Here's how the part is built. I have some questions about the finished solid (model axes, mm). A direction names the side the tool comes from. Give positions to 0.01 mm unless a question says otherwise; leave off trailing zeros. Write each loop counter-clockwise with the first axis right and the second up, starting at its lowest first coordinate (ties: lowest second). Pieces come first, ordered by that corner, then holes. Notation, with made-up numbers: (70, 34) - (95, 34) arc R27 ccw to (95, 53) - close; hole circle Ø1 at (80.25, 78.25). An arc over 180 degrees is marked (long way). Use one line per item in the form item = value. Start each with the question number.
from build123d import *

# Parameters (mm, degrees)
SKETCH1_W           = 40
SKETCH1_H           = 40
BOSS_EXTRUDE1_DEPTH = 50
SKETCH2_W           = 35
SKETCH2_H           = 35
CUT_EXTRUDE1_DEPTH  = 76.498344353
CUT_EXTRUDE2_DEPTH  = 76.498344353


with BuildPart() as part:
    # Sketch1 → Boss-Extrude1 (new body)
    with BuildSketch(Plane(origin=(0, 0, 0), x_dir=(1, 0, 0), z_dir=(0, 1, 0))):
        with Locations((20, 20)):
            Rectangle(SKETCH1_W, SKETCH1_H)
    extrude(amount=BOSS_EXTRUDE1_DEPTH)

    # Sketch2 → Cut-Extrude1 (cut, through all)
    with BuildSketch(Plane.XZ):
        with Locations((20, -20)):
            Rectangle(SKETCH2_W, SKETCH2_H)
    extrude(amount=-CUT_EXTRUDE1_DEPTH, mode=Mode.SUBTRACT)

    # Sketch3 → Cut-Extrude2 (cut, through all)
    with BuildSketch(Plane.ZY):
        Polygon((-40, 0), (0, 0), (-40, 14.558809371), align=None)
        Polygon((-40, 50), (0, 35.441190629), (0, 50), align=None)
    extrude(amount=-CUT_EXTRUDE2_DEPTH, mode=Mode.SUBTRACT)


solid = part.part
1. I want a section at A-A, the plane x = 5. List the corners of the cut face in (y, z) for me, then the cut area to 3 significant figures.
2. For faces 1 (the face through (37.5, 25, -20)), 2 (the face through (20, 32, -40)), which set-ups out of +Z, -Z, +X, -X, +Y, -Y let a thin tool reach every point of the face, with its end or its side?
3. I want a section at D-D, the plane y = 45.5. List the corners of the cut face in (x, z) for me.
4. Please list where these lines run through material, in increasing order: line 1 (X direction, y = 20, z = -8); line 2 (Z direction, x = 10.5, y = 23); line 3 (Z direction, x = 7, y = 5).
5. We'd pull the mould along X, two halves only. Please class faces 3 (the face through (2.129, 42.755, -20.093)), 4 (the face through (2.5, 25, -20)), 5 (the face through (40, 25, -20)): pulls with the +X half, pulls with the -X half, needs draft (parallel to the pull), parting line crosses it, or undercut.
6. For P1, Ø5, axis at y = 18, z = -28, coming from the -X side; P2, Ø5, axis at x = 7.5, z = -4.5, coming from the +Y side, each with a flat end and sliding along its axis, tell me the tip position at first contact or that it passes through.
7. I want a section at B-B, the plane y = 20. List the corners of the cut face in (x, z) for me, then the cut area to 3 significant figures.
8. I want a section at C-C, the plane z = -27.5. List the corners of the cut face in (x, y) for me, then the cut area to 3 significant figures.
Result sheet:
q1.outline = (0, 0) - (0.91, -2.5) - (36.35, -2.5) - (35.44, 0) - close; (13.65, -37.5) - (14.56, -40) - (50, -40) - (49.09, -37.5) - close
q1.area = 177 mm2
q2.face_1 = +Y, -Y
q2.face_2 = -Z, +X, -X, +Y, -Y
q3.outline = (0, -40) - (40, -40) - (40, -27.64) - (37.5, -27.64) - (37.5, -37.5) - (2.5, -37.5) - (2.5, -27.64) - (0, -27.64) - close
q4.line_1 = 0 to 2.5, 37.5 to 40
q4.line_2 = -40 to -37.5, -2.5 to 0
q4.line_3 = -2.5 to 0
q5.face_3 = needs draft
q5.face_4 = undercut
q5.face_5 = pulls with the +X half
q6.P1 = 0
q6.P2 = 36.35
q7.outline = (0, -40) - (40, -40) - (40, 0) - (0, 0) - close; hole (2.5, -37.5) - (37.5, -37.5) - (37.5, -2.5) - (2.5, -2.5) - close
q7.area = 375 mm2
q8.outline = (0, 10.01) - (2.5, 10.01) - (2.5, 45.45) - (0, 45.45) - close; (37.5, 10.01) - (40, 10.01) - (40, 45.45) - (37.5, 45.45) - close
q8.area = 177 mm2
